from build123d import *

# Parameters (mm, degrees)
F0_W      = 50.8
F0_H      = 25.4
F1_DEPTH  = 12.7
F2_R      = 12.7
F3_DEPTH  = 12.7
F4_R      = 12.7
F5_DEPTH  = 12.7
F6_W      = 25.4
F6_H      = 25.4
F7_DEPTH  = 19.05
F8_R      = 12.7
F9_DEPTH  = 25.4
F10_R     = 6.35
F11_DEPTH = 25.4
F12_R     = 6.35
F13_DEPTH = 12.7


with BuildPart() as f1:
    # F0 (on Top) → F1 (new body)
    with BuildSketch(Plane.XY):
        with Locations((25.4, 12.7)):
            Rectangle(F0_W, F0_H)
    extrude(amount=F1_DEPTH)

    # F2 (on face) → F3 (join)
    with BuildSketch(Plane.XY.offset(12.7)):
        with Locations((0, 12.7)):
            Circle(F2_R)
    extrude(amount=-F3_DEPTH)

    # F4 (on face) → F5 (join)
    with BuildSketch(Plane.XY.offset(12.7)):
        with Locations((50.8, 12.7)):
            Circle(F4_R)
    extrude(amount=-F5_DEPTH)

    # F6 (on face) → F7 (join)
    with BuildSketch(Plane.XY.offset(12.7)):
        with Locations((25.4, 12.7)):
            Rectangle(F6_W, F6_H)
    extrude(amount=F7_DEPTH)

    # F8 (on face) → F9 (join)
    with BuildSketch(Plane(origin=(12.7, 0, 0), x_dir=(0, -1, 0), z_dir=(-1, 0, 0))):
        with Locations((-12.7, 31.75)):
            Circle(F8_R)
    extrude(amount=-F9_DEPTH)

    # F10 (on face) → F11 (cut)
    with BuildSketch(Plane(origin=(12.7, 0, 0), x_dir=(0, -1, 0), z_dir=(-1, 0, 0))):
        with Locations((-12.7, 31.75)):
            Circle(F10_R)
    extrude(amount=-F11_DEPTH, mode=Mode.SUBTRACT)

    # F12 (on face) → F13 (cut)
    with BuildSketch(Plane.XY.offset(12.7)):
        with Locations((50.8, 12.7)):
            Circle(F12_R)
        with Locations((0, 12.7)):
            Circle(F12_R)
    extrude(amount=-F13_DEPTH, mode=Mode.SUBTRACT)


solid = f1.part
Verification items for the finished model (mm, model axes). A direction names the side the tool comes from. Coordinates: 2 decimals unless noted, no trailing zeros. Loops run counter-clockwise (first coordinate to the right, second up) from the corner with the lowest first, then second, coordinate; pieces in that order, holes last. Notation, with made-up numbers: (20, -26) -> (77, -26) arc R23 cw to (77, -11) -> close; hole circle Ø1 at (34.5, 9). An arc over 180 degrees is marked (long way). Answer as CSV lines item,"result".
1) Cross-section at C-C, the plane x = 52. Record the cut outline in (y, z), then the cut area to 3 significant figures.
Found:
outline,"(0.06, 0) -> (6.46, 0) -> (6.46, 12.7) -> (0.06, 12.7) -> close; (18.94, 0) -> (25.34, 0) -> (25.34, 12.7) -> (18.94, 12.7) -> close"
area,"163 mm2"
2) Cross-section at B-B, the plane z = 5. Record the cut outline in (x, y).
Found:
outline,"(0, 0) -> (50.8, 0) arc R12.7 ccw to (50.8, 25.4) -> (0, 25.4) arc R12.7 ccw to start; hole circle Ø12.7 at (0, 12.7); hole circle Ø12.7 at (50.8, 12.7)"
3) Depth check by flat-ended pin: pin 1 (5 mm diameter, centred on x = 19, z = 13.5, fed in from -Y); pin 2 (2 mm diameter, centred on y = 9.5, z = 10, fed in from +X); pin 3 (4 mm diameter, centred on y = 21, z = 24.5, fed in from +X); pin 4 (12.5 mm diameter, centred on y = 12.5, z = 34.5, fed in from -X). Enter the tip coordinate at first touch or a pass-through.
Found:
pin 1,"stops at y = 0"
pin 2,"stops at x = 63.31"
pin 3,"stops at x = 38.1"
pin 4,"stops at x = 12.7"
4) Thickness scan on L1, parallel to Y at x = 0, z = 5.5; L2, parallel to X at y = 18.5, z = 4; L3, parallel to Z at x = 27.25, y = 12.7. Record the ranges inside material, lowest first. Write a range as from..to.
Found:
L1,"y = 0..6.35, 19.05..25.4"
L2,"x = -11.3..-2.59, 2.59..48.21, 53.39..62.1"
L3,"z = 0..25.4, 38.1..44.45"
5) Release check for a two-part mould opening along Z. For faces 1 (the cylindrical face through (25.222, 6.643, 33.657)), 2 (the flat face through (3, 19, 12.7)), 3 (the flat face through (25, 0, 12)) record: +Z half, -Z half, draft (parallel to the pull), parting line (faces both ways), or undercut.
Found:
face 1,"undercut"
face 2,"+Z half"
face 3,"draft"
6) Cross-section at D-D, the plane y = 15. Record the cut outline in (x, z).
Found:
outline,"(-12.49, 0) -> (-5.92, 0) -> (-5.92, 12.7) -> (-12.49, 12.7) -> close; (5.92, 0) -> (44.88, 0) -> (44.88, 12.7) -> (38.1, 12.7) -> (38.1, 25.83) -> (12.7, 25.83) -> (12.7, 12.7) -> (5.92, 12.7) -> close; (12.7, 37.67) -> (38.1, 37.67) -> (38.1, 44.24) -> (12.7, 44.24) -> close; (56.72, 0) -> (63.29, 0) -> (63.29, 12.7) -> (56.72, 12.7) -> close"
7) Tool access check on faces 4 (the flat face through (45, 16, 12.7)), 5 (the cylindrical face through (3.414, 18.054, 6.439)), 6 (the flat face through (12.7, 13, 25)). Record the directions out of +Z, -Z, +X, -X, +Y, -Y that give a thin tool (end or side, any length) a straight path to the whole face; none if there is none.
Found:
face 4,"+Z, +X, +Y, -Y"
face 5,"+Z, -Z"
face 6,"+Z, -X, +Y, -Y"
8) Cross-section at A-A, the plane x = 27.5. Record the cut outline in (y, z), then the cut area to 3 significant figures.
Found:
outline,"(0, 0) -> (25.4, 0) -> (25.4, 31.75) arc R12.7 ccw to (0, 31.75) -> close; hole circle Ø12.7 at (12.7, 31.75)"
area,"933 mm2"
